Verification items for the finished model (mm, model axes). A direction names the side the tool comes from. Round coordinates to 2 decimals unless told otherwise and drop trailing zeros. Write each loop counter-clockwise with the first axis right and the second up, starting at its lowest first coordinate (ties: lowest second). Pieces come first, ordered by that corner, then holes. Notation, with made-up numbers: M -39.5,-16.75 L 1.5,-16.75 A34 ccw 1.5,22.25 Z; hole C -33,-28 d1. An arc over 180 degrees is marked long. One line per item, written item: value. Start each with the question number.
from build123d import *

# Parameters (mm, degrees)
SKETCH_1_W          = 50.5
SKETCH_1_H          = 20
EXTRUDE_1_DEPTH     = 1
SKETCH_2_W          = 1
SKETCH_2_H          = 20
EXTRUDE_2_DEPTH     = 40
CUT_EXTRUDE_2_DEPTH = 100
SKETCH_4_R          = 0.5
CUT_EXTRUDE_3_DEPTH = 66.812232905
CUT_EXTRUDE_4_REACH = 51.179
SKETCH_5_R          = 1.5


with BuildPart() as part:
    # 草图1 → 凸台-拉伸1 (new body)
    with BuildSketch(Plane.XY):
        Rectangle(SKETCH_1_W, SKETCH_1_H)
    extrude(amount=EXTRUDE_1_DEPTH)

    # 草图2 → 凸台-拉伸2 (add)
    with BuildSketch(Plane.XY.offset(1)):
        with Locations((-24.75, 0)):
            Rectangle(SKETCH_2_W, SKETCH_2_H)
        with Locations((24.75, 0)):
            Rectangle(SKETCH_2_W, SKETCH_2_H)
    extrude(amount=EXTRUDE_2_DEPTH)

    # 草图3 → 切除-拉伸2 (cut)
    with BuildSketch(Plane.ZY.offset(25.25)):
        with BuildLine():
            Line((31, -10), (41, -10))
            Line((41, -10), (41, 0))
            ThreePointArc((41, 0), (38.071067812, -7.071067812), (31, -10))
        make_face()
        with BuildLine():
            ThreePointArc((31, 10), (38.071067812, 7.071067812), (41, 0))
            Line((41, 0), (41, 10))
            Line((41, 10), (31, 10))
        make_face()
    extrude(amount=-CUT_EXTRUDE_2_DEPTH, mode=Mode.SUBTRACT)

    # 草图4 → 切除-拉伸3 (cut, through all)
    with BuildSketch(Plane(origin=(25.25, 0, 0), x_dir=(0, 0, -1), z_dir=(1, 0, 0))):
        with Locations((-39, 0)):
            Circle(SKETCH_4_R)
        with Locations((-31, 8)):
            Circle(SKETCH_4_R)
        with Locations((-23, 0)):
            Circle(SKETCH_4_R)
        with Locations((-31, -8)):
            Circle(SKETCH_4_R)
    extrude(amount=-CUT_EXTRUDE_3_DEPTH, mode=Mode.SUBTRACT)

    # 草图5 → 切除-拉伸4 (cut, up to next)
    with BuildSketch(Plane(origin=(0, 0, 0), x_dir=(-1, 0, 0), z_dir=(0, 0, -1)), mode=Mode.PRIVATE) as cut_extrude_4_sk1:
        with Locations((-5, 5)):
            Circle(SKETCH_5_R)
    cut_extrude_4_tool1 = extrude(cut_extrude_4_sk1.sketch, amount=-CUT_EXTRUDE_4_REACH, mode=Mode.PRIVATE) & part.part
    # 草图5 → 切除-拉伸4 (cut, up to next)
    with BuildSketch(Plane(origin=(0, 0, 0), x_dir=(-1, 0, 0), z_dir=(0, 0, -1)), mode=Mode.PRIVATE) as cut_extrude_4_sk2:
        with Locations((-5, -5)):
            Circle(SKETCH_5_R)
    cut_extrude_4_tool2 = extrude(cut_extrude_4_sk2.sketch, amount=-CUT_EXTRUDE_4_REACH, mode=Mode.PRIVATE) & part.part
    # 草图5 → 切除-拉伸4 (cut, up to next)
    with BuildSketch(Plane(origin=(0, 0, 0), x_dir=(-1, 0, 0), z_dir=(0, 0, -1)), mode=Mode.PRIVATE) as cut_extrude_4_sk3:
        with Locations((5, 5)):
            Circle(SKETCH_5_R)
    cut_extrude_4_tool3 = extrude(cut_extrude_4_sk3.sketch, amount=-CUT_EXTRUDE_4_REACH, mode=Mode.PRIVATE) & part.part
    # 草图5 → 切除-拉伸4 (cut, up to next)
    with BuildSketch(Plane(origin=(0, 0, 0), x_dir=(-1, 0, 0), z_dir=(0, 0, -1)), mode=Mode.PRIVATE) as cut_extrude_4_sk4:
        with Locations((5, -5)):
            Circle(SKETCH_5_R)
    cut_extrude_4_tool4 = extrude(cut_extrude_4_sk4.sketch, amount=-CUT_EXTRUDE_4_REACH, mode=Mode.PRIVATE) & part.part
    add(cut_extrude_4_tool1.solids().sort_by_distance((5, 5, 0))[0], mode=Mode.SUBTRACT)
    add(cut_extrude_4_tool2.solids().sort_by_distance((5, -5, 0))[0], mode=Mode.SUBTRACT)
    add(cut_extrude_4_tool3.solids().sort_by_distance((-5, 5, 0))[0], mode=Mode.SUBTRACT)
    add(cut_extrude_4_tool4.solids().sort_by_distance((-5, -5, 0))[0], mode=Mode.SUBTRACT)


solid = part.part
1) Gauge pin test, flat end, axial feed: pin 1 Ø4 at (x, y) = (-5, 5) entering from +Z. Record the tip position at first contact, or that the pin passes through.
2) Cross-section at D-D (y = -1.25). Record the boundary of the cut face in (x, z), then the cut area to 3 significant figures.
3) Thickness scan on line 1 (X direction, y = 8.5, z = 35); line 2 (Z direction, x = -21.5, y = -2.75). Record the ranges inside material, lowest first.
4) Cross-section at B-B (z = 11). Record the boundary of the cut face in (x, y), then the cut area to 3 significant figures.
5) Cross-section at C-C (y = 5). Record the boundary of the cut face in (x, z).
6) Access from +Z, -Z, +X, -X, +Y, -Y to the whole of each face (thin tool, end or side, straight path). Record for faces 5 (the flat face through (24.25, 0, 21)), 6 (the cylindrical face through (-6.386, 4.425, 0.493)).
7) Cross-section at A-A (x = -5). Record the boundary of the cut face in (y, z), then the cut area to 3 significant figures.
8) Mould release check, pull along X, two halves, no side actions. Record for faces 1 (the flat face through (25.25, 0, 20)), 2 (the flat face through (0, 0, 0)), 3 (the flat face through (-25.25, 0, 20)), 4 (the flat face through (-24.25, 0, 21)): pulls with the +X half, pulls with the -X half, needs draft (parallel to the pull), parting line crosses it, or undercut.
Results below:
1. pin 1: stops at z = 1
2. outline: M -25.25,0 L 25.25,0 L 25.25,40.92 L 24.25,40.92 L 24.25,1 L -24.25,1 L -24.25,40.92 L -25.25,40.92 Z
2. area: 130 mm²
3. line 1: x = -25.25 to -24.25, 24.25 to 25.25
3. line 2: z = 0 to 1
4. outline: M -25.25,-10 L -24.25,-10 L -24.25,10 L -25.25,10 Z; M 24.25,-10 L 25.25,-10 L 25.25,10 L 24.25,10 Z
4. area: 40.0 mm²
5. outline: M -25.25,0 L -6.5,0 L -6.5,1 L -24.25,1 L -24.25,39.66 L -25.25,39.66 Z; M -3.5,0 L 3.5,0 L 3.5,1 L -3.5,1 Z; M 6.5,0 L 25.25,0 L 25.25,39.66 L 24.25,39.66 L 24.25,1 L 6.5,1 Z
6. face 5: +Z, +Y, -Y
6. face 6: +Z, -Z
7. outline: M -10,0 L -6.5,0 L -6.5,1 L -10,1 Z; M -3.5,0 L 3.5,0 L 3.5,1 L -3.5,1 Z; M 6.5,0 L 10,0 L 10,1 L 6.5,1 Z
7. area: 14.0 mm²
8. face 1: pulls with the +X half
8. face 2: needs draft
8. face 3: pulls with the -X half
8. face 4: undercut
